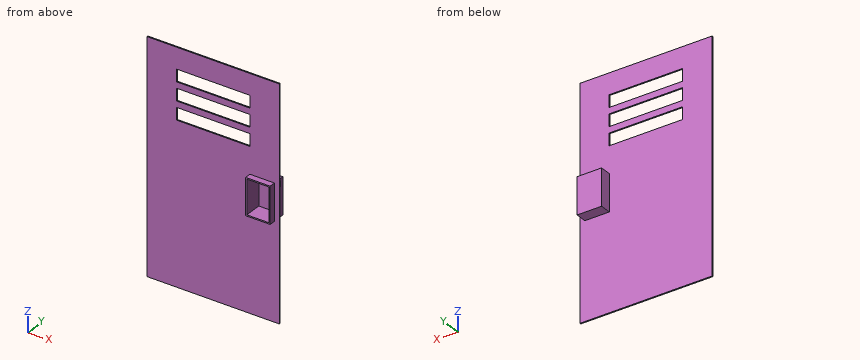
from build123d import *

# Parameters (mm, degrees)
F0_W          = 274.32
F0_H          = 477.52
F1_DEPTH      = 2.54
F2_W          = 152.4
F2_H          = 25.4
F3_W          = 152.4
F3_H          = 25.4
F4_W          = 152.4
F4_H          = 25.4
F5_DEPTH      = 25.4
F6_W          = 45.72
F6_H          = 76.2
F7_DEPTH      = 25.4
F8_W          = 50.8
F8_H          = 76.2
F9_DEPTH      = 12.7
F9_DEPTH_BACK = 25.4
F10_T         = 2.54
F10_T3_DEPTH  = 7.4696609569
F10_T5_DEPTH  = 81.28
F10_T7_DEPTH  = 55.88
F10_T9_DEPTH  = 7.7703390431
F10_T11_DEPTH = 7.62
F11_W         = 13.208
F11_H         = 12.7
F12_DEPTH     = 25.4


# Not quite as in the source:
# - a shell that OpenCascade refuses in one call is made with other operations: the cavity is built on its own and cut out


with BuildPart() as f1:
    # F0 (on Front) → F1 (new body)
    with BuildSketch(Plane.XZ):
        Rectangle(F0_W, F0_H)
    extrude(amount=F1_DEPTH)

    # F2 (on face) + F3 (on face) + F4 (on face) → F5 (cut)
    with BuildSketch(Plane.XZ.offset(2.54)):
        with Locations((0, 182.5210501183)):
            Rectangle(F2_W, F2_H)
    with BuildSketch(Plane.XZ.offset(2.54)):
        with Locations((0, 144.4210501183)):
            Rectangle(F3_W, F3_H)
    with BuildSketch(Plane.XZ.offset(2.54)):
        with Locations((0, 106.3210501183)):
            Rectangle(F4_W, F4_H)
    extrude(amount=-F5_DEPTH, mode=Mode.SUBTRACT)

    # F6 (on face) → F7 (cut)
    with BuildSketch(Plane.XZ.offset(2.54)):
        with Locations((101.6, 0)):
            Rectangle(F6_W, F6_H)
    extrude(amount=-F7_DEPTH, mode=Mode.SUBTRACT)

    # F8 (on face) → F9 (join, two sides)
    with BuildSketch(Plane.XZ.offset(2.54)) as f9_sk:
        with Locations((101.4496609569, 0.1478558406)):
            Rectangle(F8_W, F8_H)
    extrude(amount=F9_DEPTH)
    extrude(f9_sk.sketch, amount=-F9_DEPTH_BACK)

    # F10: shell of thickness 2.54, made by hand


with BuildPart() as f10_core1:
    # F10_t2: copy of F1
    add(f1.part)

    # the walls: a layer under each face that stays
    f10_faces = [f10_core1.faces().sort_by_distance(p)[0] for p in [
        (0, -1.27, 238.76),
        (137.16, -1.27, 0),
        (-137.16, -1.27, 0),
        (0, 0, 0),
        (0, -2.54, 0),
        (0, -1.27, -238.76),
        (101.6, -1.27, -38.1),
        (124.46, -1.27, -38.0260720797),
        (101.4496609569, 3.81, -37.9521441594),
        (126.8496609569, 11.43, 0.1478558406),
        (101.4496609569, 11.43, 38.2478558406),
        (76.0496609569, 11.43, 0.1478558406),
        (78.74, -1.27, -38.0260720797),
        (-76.2, -1.27, 106.3210501183),
        (0, -1.27, 119.0210501183),
        (0, -1.27, 93.6210501183),
        (76.2, -1.27, 106.3210501183),
        (0, -1.27, 131.7210501183),
        (-76.2, -1.27, 144.4210501183),
        (76.2, -1.27, 144.4210501183),
        (0, -1.27, 157.1210501183),
        (0, -1.27, 169.8210501183),
        (-76.2, -1.27, 182.5210501183),
        (76.2, -1.27, 182.5210501183),
        (0, -1.27, 195.2210501183),
        (126.8496609569, -8.89, 0.1478558406),
        (101.4496609569, -8.89, 38.2478558406),
        (76.0496609569, -8.89, 0.1478558406),
        (101.4496609569, 22.86, 0.1478558406),
    ]]
    thicken(f10_faces, amount=-F10_T, mode=Mode.SUBTRACT)

    # F10_s4 → F10_t3 (cut)
    with BuildSketch(Plane.YZ.offset(121.92)):
        Polygon((0.0254, -37.9775441594), (-2.54, -37.9521441594), (-2.54, -35.4121441594), (0, -35.4121441594), align=None)
        Polygon((-2.5654, -37.9775441594), (0, -37.9521441594), (0, -35.4121441594), (-2.54, -35.4121441594), align=None)
    extrude(amount=F10_T3_DEPTH, mode=Mode.SUBTRACT)

    # F10_s6 → F10_t5 (cut)
    with BuildSketch(Plane.XY.offset(-40.4921441594)):
        Polygon((126.8750609569, 0.0254), (126.8496609569, -2.54), (124.3096609569, -2.54), (124.3096609569, 0), align=None)
        Polygon((76.0242609569, 0.0254), (76.0496609569, -2.54), (78.5896609569, -2.54), (78.5896609569, 0), align=None)
        Polygon((126.8750609569, -2.5654), (126.8496609569, 0), (124.3096609569, 0), (124.3096609569, -2.54), align=None)
        Polygon((76.0242609569, -2.5654), (76.0496609569, 0), (78.5896609569, 0), (78.5896609569, -2.54), align=None)
    extrude(amount=F10_T5_DEPTH, mode=Mode.SUBTRACT)

    # F10_s8 → F10_t7 (cut)
    with BuildSketch(Plane.YZ.offset(73.5096609569)):
        Polygon((0.0254, 38.2732558406), (-2.54, 38.2478558406), (-2.54, 35.7078558406), (0, 35.7078558406), align=None)
        Polygon((-2.5654, 38.2732558406), (0, 38.2478558406), (0, 35.7078558406), (-2.54, 35.7078558406), align=None)
    extrude(amount=F10_T7_DEPTH, mode=Mode.SUBTRACT)

    # F10_s10 → F10_t9 (cut)
    with BuildSketch(Plane.YZ.offset(73.5096609569)):
        Polygon((0.0254, -37.9775441594), (-2.54, -37.9521441594), (-2.54, -35.4121441594), (0, -35.4121441594), align=None)
        Polygon((-2.5654, -37.9775441594), (0, -37.9521441594), (0, -35.4121441594), (-2.54, -35.4121441594), align=None)
    extrude(amount=F10_T9_DEPTH, mode=Mode.SUBTRACT)

    # F10_s12 → F10_t11 (cut)
    with BuildSketch(Plane.XZ.offset(-2.54)):
        Polygon((124.4346, -38.0746), (124.46, -40.64), (127, -40.64), (127, -38.1), align=None)
        Polygon((78.7654, -38.0746), (78.74, -40.64), (76.2, -40.64), (76.2, -38.1), align=None)
        Polygon((124.4346, -37.9775441594), (127, -37.9521441594), (127, -35.4121441594), (124.46, -35.4121441594), align=None)
        Polygon((78.7654, -37.9775441594), (78.74, -35.4121441594), (76.2, -35.4121441594), (76.2, -37.9521441594), align=None)
        Polygon((-76.1746, 93.6464501183), (-78.74, 93.6210501183), (-78.74, 91.0810501183), (-76.2, 91.0810501183), align=None)
        Polygon((-76.1746, 118.9956501183), (-78.74, 119.0210501183), (-78.74, 121.5610501183), (-76.2, 121.5610501183), align=None)
        Polygon((76.1746, 118.9956501183), (76.2, 121.5610501183), (78.74, 121.5610501183), (78.74, 119.0210501183), align=None)
        Polygon((76.1746, 93.6464501183), (76.2, 91.0810501183), (78.74, 91.0810501183), (78.74, 93.6210501183), align=None)
        Polygon((76.1746, 131.7464501183), (76.2, 129.1810501183), (78.74, 129.1810501183), (78.74, 131.7210501183), align=None)
        Polygon((-76.1746, 131.7464501183), (-76.2, 129.1810501183), (-78.74, 129.1810501183), (-78.74, 131.7210501183), align=None)
        Polygon((-76.1746, 157.0956501183), (-78.74, 157.1210501183), (-78.74, 159.6610501183), (-76.2, 159.6610501183), align=None)
        Polygon((76.1746, 157.0956501183), (78.74, 157.1210501183), (78.74, 159.6610501183), (76.2, 159.6610501183), align=None)
        Polygon((76.1746, 169.8464501183), (76.2, 167.2810501183), (78.74, 167.2810501183), (78.74, 169.8210501183), align=None)
        Polygon((-76.1746, 169.8464501183), (-76.2, 167.2810501183), (-78.74, 167.2810501183), (-78.74, 169.8210501183), align=None)
        Polygon((-76.1746, 195.1956501183), (-78.74, 195.2210501183), (-78.74, 197.7610501183), (-76.2, 197.7610501183), align=None)
        Polygon((76.1746, 195.1956501183), (78.74, 195.2210501183), (78.74, 197.7610501183), (76.2, 197.7610501183), align=None)
    extrude(amount=F10_T11_DEPTH, mode=Mode.SUBTRACT)


with BuildPart() as f1_1:
    add(f1.part)

    # what is left inside the walls is the cavity
    f10_cavity = [f10_core1.part.solids().sort_by_distance(p)[0] for p in [
        (101.449661, -15.2146, -11.705477),
    ]]
    add(f10_cavity, mode=Mode.SUBTRACT)

    # F11 (on face) → F12 (cut)
    with BuildSketch(Plane.YZ.offset(126.8496609569)):
        with Locations((9.7576510161, 28.402006929)):
            Rectangle(F11_W, F11_H)
    extrude(amount=-F12_DEPTH, mode=Mode.SUBTRACT)


solid = f1_1.part
For this review, take the finished solid that the model builds, in its own axes (mm). Round coordinates to 2 decimals unless told otherwise and drop trailing zeros. Write each loop counter-clockwise with the first axis right and the second up, starting at its lowest first coordinate (ties: lowest second). Pieces come first, ordered by that corner, then holes. Notation, with made-up numbers: (3.25, 38) - (15.25, 38) arc R20 ccw to (15.25, 76) - close; hole circle Ø3 at (-36, -0.5). An arc over 180 degrees is marked (long way). Write item = value, one per line. Start each with the question number.
1. Consider section A-A on x = 103.5. State the section outline as (y, z) points, plus the area to 3 significant figures.
2. Consider section B-B on x = -36.5. State the section outline as (y, z) points.
3. Consider section C-C on z = 105. State the section outline as (x, y) points, plus the area to 3 significant figures.
4. Consider section D-D on y = 8. State the section outline as (x, z) points.
5. Wall thickness on L1, parallel to Z at x = -43, y = -1; L2, parallel to Z at x = 105, y = -10; L3, parallel to X at y = -6, z = 22: over which ranges is each line inside the solid? List them lowest first.
6. For pin 1 Ø4 at (x, y) = (113.5, -7) entering from +Z; pin 2 Ø4 at (x, z) = (-13.5, -69.5) entering from -Y; pin 3 Ø6 at (x, z) = (-44.5, -75.5) entering from +Y, all flat-tipped, find the tip position at first contact; note any pin that passes through.
Evaluation:
q1.outline = (-15.24, -37.95) - (22.86, -37.95) - (22.86, 38.25) - (0, 38.25) - (0, 238.76) - (-2.54, 238.76) - (-2.54, 38.25) - (-15.24, 38.25) - (-15.24, 35.71) - (20.32, 35.71) - (20.32, -35.41) - (-15.24, -35.41) - close; (-2.54, -238.76) - (0, -238.76) - (0, -38.1) - (-2.54, -38.1) - close
q1.area = 1,390 mm2
q2.outline = (-2.54, -238.76) - (0, -238.76) - (0, 93.62) - (-2.54, 93.62) - close; (-2.54, 119.02) - (0, 119.02) - (0, 131.72) - (-2.54, 131.72) - close; (-2.54, 157.12) - (0, 157.12) - (0, 169.82) - (-2.54, 169.82) - close; (-2.54, 195.22) - (0, 195.22) - (0, 238.76) - (-2.54, 238.76) - close
q3.outline = (-137.16, -2.54) - (-76.2, -2.54) - (-76.2, 0) - (-137.16, 0) - close; (76.2, -2.54) - (137.16, -2.54) - (137.16, 0) - (76.2, 0) - close
q3.area = 310 mm2
q4.outline = (76.05, -37.95) - (126.85, -37.95) - (126.85, 22.05) - (124.31, 22.05) - (124.31, -35.41) - (78.59, -35.41) - (78.59, 35.71) - (124.31, 35.71) - (124.31, 34.75) - (126.85, 34.75) - (126.85, 38.25) - (76.05, 38.25) - close
q5.L1 = -238.76 to 93.62, 119.02 to 131.72, 157.12 to 169.82, 195.22 to 238.76
q5.L2 = -37.95 to -35.41, 35.71 to 38.25
q5.L3 = 76.05 to 78.59, 124.31 to 126.85
q6.pin_1 = 38.25
q6.pin_2 = -2.54
q6.pin_3 = 0
